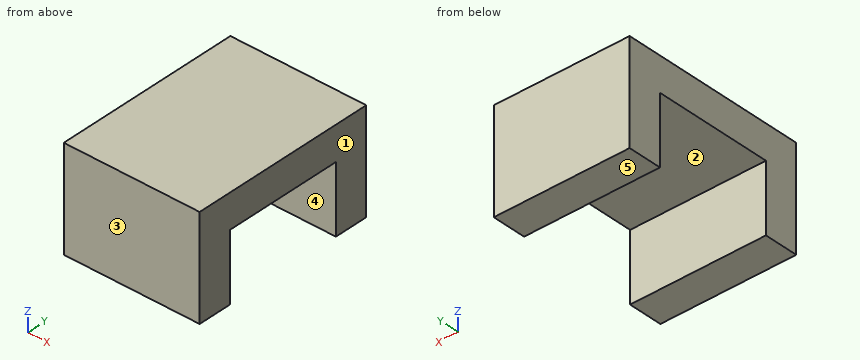
from build123d import *

# Parameters (mm, degrees)
F0_W     = 40
F0_H     = 35
F1_DEPTH = 30
F0_H_2   = 10
F2_DEPTH = 30
F3_W     = 40
F3_H     = 35
F4_DEPTH = 20


with BuildPart() as f1:
    # F0 (on Top) → F1 (new body)
    with BuildSketch(Plane.XY):
        with Locations((-0.33484, 0.644105)):
            Rectangle(F0_W, F0_H)
    extrude(amount=F1_DEPTH)

    # F0 (on Top) → F2 (join)
    with BuildSketch(Plane.XY):
        with Locations((-0.33484, 23.144105)):
            Rectangle(F0_W, F0_H_2)
        with Locations((-0.33484, 0.644105)):
            Rectangle(F0_W, F0_H)
        with Locations((-0.33484, -21.855895)):
            Rectangle(F0_W, F0_H_2)
    extrude(amount=F2_DEPTH)

    # F3 (on face) → F4 (cut)
    with BuildSketch(Plane(origin=(0, 0, 0), x_dir=(1, 0, 0), z_dir=(0, 0, -1))):
        with Locations((-0.33484, -0.644105)):
            Rectangle(F3_W, F3_H)
    extrude(amount=-F4_DEPTH, mode=Mode.SUBTRACT)


solid = f1.part
Geometry: final body of the model. Coordinates: model frame, mm. Face numbers are marked on the shaded views. A direction names the side the tool comes from. Round coordinates to 2 decimals unless told otherwise and drop trailing zeros. Order: outer loops, then holes, each group sorted by start corner. A loop starts at its lowest first (then second) coordinate and runs counter-clockwise, first axis right, second up.
Q1. Section C-C, the plane y = -2.5. Output: boundary loops of the cut face in (x, z).
Result sheet:
outline: (-20.33, 20) - (19.67, 20) - (19.67, 30) - (-20.33, 30) - close
Q2. Access query for the marked faces 4 and 5. Directions: +Z, -Z, +X, -X, +Y, -Y. A direction counts if a zero-diameter tool reaches every point of the face in a straight line with its end or side. Return the directions, or none.
Result sheet:
face 4: -Z, +X, -X
face 5: -Z, +X, -X, +Y, -Y
Q3. Section B-B, the plane x = 9. Output: boundary loops of the cut face in (y, z), and give its area (3 significant figures).
Result sheet:
outline: (-26.86, 0) - (-16.86, 0) - (-16.86, 20) - (18.14, 20) - (18.14, 0) - (28.14, 0) - (28.14, 30) - (-26.86, 30) - close
area: 950 mm2
Q4. Section A-A, the plane z = 2. Output: boundary loops of the cut face in (x, y).
Result sheet:
outline: (-20.33, -26.86) - (19.67, -26.86) - (19.67, -16.86) - (-20.33, -16.86) - close; (-20.33, 18.14) - (19.67, 18.14) - (19.67, 28.14) - (-20.33, 28.14) - close
Q5. Pin query (flat end, axial travel): pin 1 (5 mm diameter, centred on x = -9.5, y = -6, fed in from -Z). Return the tip coordinate at first contact, or that it passes through.
Result sheet:
pin 1: stops at z = 20
Q6. Mould query, pull axis Y, two halves, no side actions, for the marked faces 1, 2 and 3. Classes: released by +Y, released by -Y, zero draft, split by the parting line, or undercut.
Result sheet:
face 1: zero draft
face 2: undercut
face 3: released by -Y
Q7. Material intervals for probe 1 along Y at (x, z) = (18, 4.25); probe 2 along Z at (x, y) = (10, 12.5), sorted ascending.
Result sheet:
probe 1: y = -26.86 to -16.86, 18.14 to 28.14
probe 2: z = 20 to 30
